Work out the finished part from the listing and answer in its coordinate system (mm). Give positions to 0.01 mm unless a question says otherwise; leave off trailing zeros. Loops run counter-clockwise (first coordinate to the right, second up) from the corner with the lowest first, then second, coordinate; pieces in that order, holes last. Notation, with made-up numbers: (61.25, -21) - (113.25, -21) arc R24 cw to (113.25, 9) - close; hole circle Ø2 at (6.25, 45.25). An arc over 180 degrees is marked (long way). One line per item, written item: value.
from build123d import *

# Parameters (mm, degrees)
IZIM2_W               = 160
IZIM2_H               = 200
TABAN_FLAN_1_DEPTH    = 8
K_ELERI_START         = -8
K_ELERI_K_R1_DEPTH    = 8
IZIM3_R               = 8.5
KES_EKSTR_ZYON1_DEPTH = 216.555097365
IZIM4_R               = 3
KES_EKSTR_ZYON2_DEPTH = 216.555097365


# Read off the part's stored shape, not the designer's step: Köşeleri kır1
# Sheet-metal steps are written as plain solids
with BuildPart() as part:
    # Çizim2 → Taban-Flanş1 (new body)
    with BuildSketch(Plane(origin=(0, 0, 0), x_dir=(1, 0, 0), z_dir=(0, 1, 0))):
        with Locations((0, -100)):
            Rectangle(IZIM2_W, IZIM2_H)
    extrude(amount=-TABAN_FLAN_1_DEPTH)

    # Köşeleri kır1 outline → Köşeleri kır1 (cut)
    with BuildSketch(Plane(origin=(0, 0, 0), x_dir=(1, 0, 0), z_dir=(0, 1, 0)).offset(K_ELERI_START)):
        with BuildLine():
            ThreePointArc((80, -196), (78.828427125, -198.828427125), (76, -200))
            Line((76, -200), (80, -200))
            Line((80, -200), (80, -196))
        make_face()
        with BuildLine():
            Line((-80, -200), (-76, -200))
            ThreePointArc((-76, -200), (-78.828427125, -198.828427125), (-80, -196))
            Line((-80, -196), (-80, -200))
        make_face()
        with BuildLine():
            ThreePointArc((76, 0), (78.828427125, -1.171572875), (80, -4))
            Line((80, -4), (80, 0))
            Line((80, 0), (76, 0))
        make_face()
        with BuildLine():
            Line((-80, 0), (-80, -4))
            ThreePointArc((-80, -4), (-78.828427125, -1.171572875), (-76, 0))
            Line((-76, 0), (-80, 0))
        make_face()
    extrude(amount=K_ELERI_K_R1_DEPTH, mode=Mode.SUBTRACT)

    # Çizim3 → Kes-Ekstrüzyon1 (cut, through all)
    with BuildSketch(Plane(origin=(0, 0, 0), x_dir=(1, 0, 0), z_dir=(0, 1, 0))):
        with Locations(Location((0, -72, 0), (0, 0, 270))):
            Circle(IZIM3_R)
    extrude(amount=-KES_EKSTR_ZYON1_DEPTH, mode=Mode.SUBTRACT)

    # Çizim4 → Kes-Ekstrüzyon2 (cut, through all)
    with BuildSketch(Plane(origin=(0, 0, 0), x_dir=(1, 0, 0), z_dir=(0, 1, 0))):
        with Locations(Location((-19, -116, 0), (0, 0, 270))):
            Circle(IZIM4_R)
        with Locations(Location((19, -116, 0), (0, 0, 270))):
            Circle(IZIM4_R)
        with Locations(Location((19, -154, 0), (0, 0, 270))):
            Circle(IZIM4_R)
        with Locations(Location((-19, -154, 0), (0, 0, 270))):
            Circle(IZIM4_R)
    extrude(amount=-KES_EKSTR_ZYON2_DEPTH, mode=Mode.SUBTRACT)


solid = part.part
1. Section A-A (x = -19) is taken. Write down the section's boundary in (y, z), and give its area (3 significant figures).
Output:
outline: (-8, 0) - (0, 0) - (0, 113) - (-8, 113) - close; (-8, 119) - (0, 119) - (0, 151) - (-8, 151) - close; (-8, 157) - (0, 157) - (0, 200) - (-8, 200) - close
area: 1,500 mm²
2. Section B-B (x = 0) is taken. Write down the section's boundary in (y, z).
Output:
outline: (-8, 0) - (0, 0) - (0, 63.5) - (-8, 63.5) - close; (-8, 80.5) - (0, 80.5) - (0, 200) - (-8, 200) - close
3. Section C-C (z = 153.5) is taken. Write down the section's boundary in (x, y), and give its area (3 significant figures).
Output:
outline: (-80, -8) - (-21.96, -8) - (-21.96, 0) - (-80, 0) - close; (-16.04, -8) - (16.04, -8) - (16.04, 0) - (-16.04, 0) - close; (21.96, -8) - (80, -8) - (80, 0) - (21.96, 0) - close
area: 1,190 mm²
4. The mould has two halves that part along X. Classify faces 1 (the cylindrical face through (17.85, -3.94, 118.77)), 2 (the flat face through (-1, 0, 99)), 3 (the cylindrical face through (-78.797, -4.056, 198.859)): released by +X, released by -X, zero draft, split by the parting line, or undercut.
Output:
face 1: undercut
face 2: zero draft
face 3: released by -X
5. Find the intervals of material crossed by line 1 along X through (y, z) = (-3.75, 116); line 2 along Z through (x, y) = (3, -3.5); line 3 along X through (y, z) = (-4.75, 66), in increasing order.
Output:
line 1: x = -80 to -22, -16 to 16, 22 to 80
line 2: z = 0 to 64.05, 79.95 to 200
line 3: x = -80 to -6.02, 6.02 to 80
6. A flat-ended cylindrical pin translates along its axis: pin 1 Ø5 at (x, z) = (19, 154) entering from -Y. Find the tip coordinate at first contact, or state that the pin passes through.
Output:
pin 1: passes through
